Build history of the part. All positions in model axes, mm. A direction names the side the tool comes from. Round coordinates to 2 decimals unless told otherwise and drop trailing zeros. Write each loop counter-clockwise with the first axis right and the second up, starting at its lowest first coordinate (ties: lowest second). Pieces come first, ordered by that corner, then holes.
Item 1: Mould opens along X. For faces 1 (the cylindrical face through (37.01, -5.44, 11.65)), 2 (the flat face through (9, -13, -9)), 3 (the cylindrical face through (11.459, -6.591, -11.327)) say: +X half, -X half, draft (parallel to the pull), parting line (faces both ways), or undercut.
Item 2: Wall check: probe 1 along X at (y, z) = (-1, 12); probe 2 along X at (y, z) = (-2.5, 17); probe 3 along Z at (x, y) = (-20, -5). Give the ranges that are in metal, low to high.
Item 3: Drop flat-ended pins along their axis: pin 1 Ø4 at (y, z) = (-2, -27.5) entering from +X; pin 2 Ø5 at (y, z) = (-4, 34.5) entering from -X; pin 3 Ø1 at (x, y) = (-16.5, -6.5) entering from -Z. Give the stop position or say it passes through.
Item 4: Band-saw the part on B-B, the plane z = 0. Write the cut outline in (x, y).
Item 5: 3-axis set-ups, long thin cutter, end or side, ignore diameter. For faces 4 (the cylindrical face through (-9.2, -6.4, 31.9)), 5 (the flat face through (3, -10, 40)): which of +Z, -Z, +X, -X, +Y, -Y reach the whole face in a straight line?
Item 6: Band-saw the part on A-A, the plane y = -5.25. Count the separate pieces of the cut face and the enclosed holes in it, then the cut area to 3 significant figures.
```python
from build123d import *

# Parameters (mm, degrees)
F0_R     = 38.8
F0_R_2   = 11.1125
F1_DEPTH = 12
F2_R     = 44.45
F2_R_2   = 38.8
F3_DEPTH = 2
F6_DEPTH = 25
F7_R     = 2
F8_SIZE  = 1
F9_DEPTH = 1


with BuildPart() as f1:
    # F0 (on Front) → F1 (new body)
    with BuildSketch(Plane.XZ):
        Circle(F0_R)
        Circle(F0_R_2, mode=Mode.SUBTRACT)
    extrude(amount=F1_DEPTH)

    # F2 (on face) → F3 (join)
    with BuildSketch(Plane.XZ.offset(12)):
        Circle(F2_R)
        Circle(F2_R_2, mode=Mode.SUBTRACT)
    extrude(amount=-F3_DEPTH)

    # F5 (on face) → F6 (cut)
    with BuildSketch(Plane.XZ.offset(12)):
        with BuildLine():
            ThreePointArc((8.7480837245, -32.6482929286), (23.9002092041, -23.9002092041), (32.6482929286, -8.7480837245))
            Line((32.6482929286, -8.7480837245), (15.5634798761, -4.1702218642))
            ThreePointArc((15.5634798761, -4.1702218642), (11.3932580119, -11.3932580119), (4.1702218642, -15.5634798761))
            Line((4.1702218642, -15.5634798761), (8.7480837245, -32.6482929286))
        make_face()
        with BuildLine():
            ThreePointArc((-32.6482929286, -8.7480837245), (-23.9002092041, -23.9002092041), (-8.7480837245, -32.6482929286))
            Line((-8.7480837245, -32.6482929286), (-4.1702218642, -15.5634798761))
            ThreePointArc((-4.1702218642, -15.5634798761), (-11.3932580119, -11.3932580119), (-15.5634798761, -4.1702218642))
            Line((-15.5634798761, -4.1702218642), (-32.6482929286, -8.7480837245))
        make_face()
        with BuildLine():
            Line((-4.1702218642, 15.5634798761), (-8.7480837245, 32.6482929286))
            ThreePointArc((-8.7480837245, 32.6482929286), (-23.9002092041, 23.9002092041), (-32.6482929286, 8.7480837245))
            Line((-32.6482929286, 8.7480837245), (-15.5634798761, 4.1702218642))
            ThreePointArc((-15.5634798761, 4.1702218642), (-11.3932580119, 11.3932580119), (-4.1702218642, 15.5634798761))
        make_face()
        with BuildLine():
            Line((15.5634798761, 4.1702218642), (32.6482929286, 8.7480837245))
            ThreePointArc((32.6482929286, 8.7480837245), (23.9002092041, 23.9002092041), (8.7480837245, 32.6482929286))
            Line((8.7480837245, 32.6482929286), (4.1702218642, 15.5634798761))
            ThreePointArc((4.1702218642, 15.5634798761), (11.3932580119, 11.3932580119), (15.5634798761, 4.1702218642))
        make_face()
    extrude(amount=-F6_DEPTH, mode=Mode.SUBTRACT)

    # F7
    f7_edges = [f1.edges().sort_by_distance(p)[0] for p in [
        (-8.748084, -6, -32.648293),
        (-4.170222, -6, -15.56348),
        (-15.56348, -6, -4.170222),
        (-32.648293, -6, -8.748084),
        (4.170222, -6, -15.56348),
        (8.748084, -6, -32.648293),
        (15.56348, -6, -4.170222),
        (32.648293, -6, -8.748084),
        (8.748084, -6, 32.648293),
        (32.648293, -6, 8.748084),
        (15.56348, -6, 4.170222),
        (4.170222, -6, 15.56348),
        (-4.170222, -6, 15.56348),
        (-15.56348, -6, 4.170222),
        (-8.748084, -6, 32.648293),
        (-32.648293, -6, 8.748084),
    ]]
    fillet(f7_edges, radius=F7_R)

    # F8
    f8_edges = [f1.edges().sort_by_distance(p)[0] for p in [
        (-38.8, 0, 0),
    ]]
    chamfer(f8_edges, length=F8_SIZE)

    # F9 (add): a face of the model
    f9_faces = [f1.faces().sort_by_distance(p)[0] for p in [
        (-10.5042580119, -12, -10.5042580119),
    ]]
    extrude(f9_faces, amount=F9_DEPTH)


solid = f1.part
```
Results:
1. face 1: parting line
1. face 2: draft
1. face 3: undercut
2. probe 1: x = -36.9 to -31.6, -10.75 to 10.75, 31.6 to 36.9
2. probe 2: x = -34.88 to -29.21, -4.6 to 4.6, 29.21 to 34.88
2. probe 3: z = -33.25 to -27.25, -5.36 to 5.36, 27.25 to 33.25
3. pin 1: stops at x = 29.24
3. pin 2: stops at x = -21.94
3. pin 3: stops at z = -35.35
4. outline: (-44.45, -13) - (-11.11, -13) - (-11.11, 0) - (-37.8, 0) - (-38.8, -1) - (-38.8, -10) - (-44.45, -10) - close; (11.11, -13) - (44.45, -13) - (44.45, -10) - (38.8, -10) - (38.8, -1) - (37.8, 0) - (11.11, 0) - close
5. face 4: +Y, -Y
5. face 5: +Y
6. separate pieces: 1
6. enclosed holes: 5
6. area: 2,510 mm2
